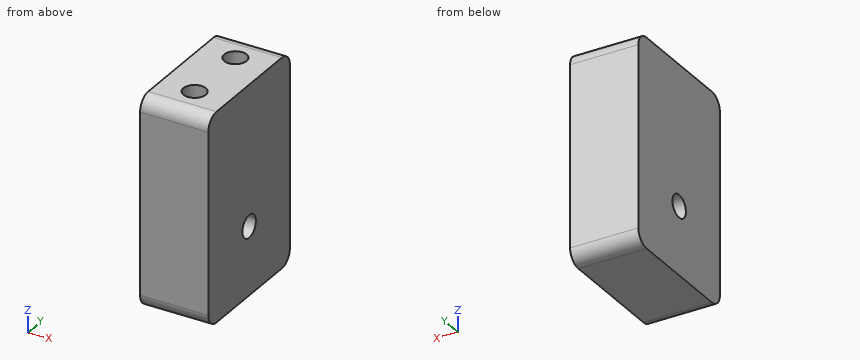
from build123d import *

# Parameters (mm, degrees)
SKETCH_1_W      = 30.5
SKETCH_1_H      = 20
SKETCH_1_R      = 1.65
EXTRUDE_1_DEPTH = 10
M4X0_7_1_D      = 3.3
M4X0_7_1_DEPTH  = 15
M4X0_7_1_TIP    = 0.991420021
FILLET_1_R      = 2


with BuildPart() as part:
    # ｽｹｯﾁ1 → ﾎﾞｽ - 押し出し1 (new body)
    with BuildSketch(Plane(origin=(0, 0, 0), x_dir=(0, 0, -1), z_dir=(1, 0, 0))):
        with Locations((15.25, 10)):
            Rectangle(SKETCH_1_W, SKETCH_1_H)
        with Locations((20.5, 10)):
            Circle(SKETCH_1_R, mode=Mode.SUBTRACT)
    extrude(amount=EXTRUDE_1_DEPTH)

    # M4x0.7 ねじ穴1
    with Locations(Plane.XY):
        with Locations((5, 5), (5, 15)):
            Hole(M4X0_7_1_D / 2, depth=M4X0_7_1_DEPTH)
            with Locations((0, 0, -(M4X0_7_1_DEPTH + M4X0_7_1_TIP / 2))):  # 118° drill point
                Cone(0, M4X0_7_1_D / 2, M4X0_7_1_TIP, mode=Mode.SUBTRACT)

    # ﾌｨﾚｯﾄ1
    fillet_1_edges = [part.edges().sort_by_distance(p)[0] for p in [
        (5, 20, 0),
        (5, 20, -30.5),
        (5, 0, -30.5),
        (5, 0, 0),
    ]]
    fillet(fillet_1_edges, radius=FILLET_1_R)


solid = part.part
The model under review builds one solid part; all positions refer to its coordinate system, in mm. Round coordinates to 2 decimals unless told otherwise and drop trailing zeros. Write each loop counter-clockwise with the first axis right and the second up, starting at its lowest first coordinate (ties: lowest second). Pieces come first, ordered by that corner, then holes. Notation, with made-up numbers: (70, 8.25) - (111, 8.25) arc R8 ccw to (111, 16.25) - close; hole circle Ø4 at (-17, 20.25). An arc over 180 degrees is marked (long way). One line per item, written item: value. Start each with the question number.
1. Consider section B-B on x = 2.5. Write out the cut boundary in (y, z), and give its area (3 significant figures).
2. To check wall thickness, follow L1, parallel to Y at x = 5, z = -10; L2, parallel to Y at x = 4, z = -20.5; L3, parallel to X at y = 15, z = -3.25. State the ranges of each line that lie inside material, in increasing order. Write a range as from..to.
3. Consider section D-D on y = 9. Write out the cut boundary in (x, z).
4. Consider section A-A on z = -20.5. Write out the cut boundary in (x, y).
5. Consider section C-C on z = -14.5. Write out the cut boundary in (x, y), and give its area (3 significant figures).
Checks:
1. outline: (0, -28.5) arc R2 ccw to (2, -30.5) - (18, -30.5) arc R2 ccw to (20, -28.5) - (20, -2) arc R2 ccw to (18, 0) - (2, 0) arc R2 ccw to (0, -2) - close; hole circle Ø3.3 at (10, -20.5)
1. area: 598 mm^2
2. L1: y = 0..3.35, 6.65..13.35, 16.65..20
2. L2: y = 0..8.35, 11.65..20
2. L3: x = 0..3.35, 6.65..10
3. outline: (0, -30.5) - (10, -30.5) - (10, -21.81) - (0, -21.81) - close; (0, -19.19) - (10, -19.19) - (10, 0) - (0, 0) - close
4. outline: (0, 0) - (10, 0) - (10, 8.35) - (0, 8.35) - close; (0, 11.65) - (10, 11.65) - (10, 20) - (0, 20) - close
5. outline: (0, 0) - (10, 0) - (10, 20) - (0, 20) - close; hole circle Ø3.3 at (5, 5); hole circle Ø3.3 at (5, 15)
5. area: 183 mm^2
